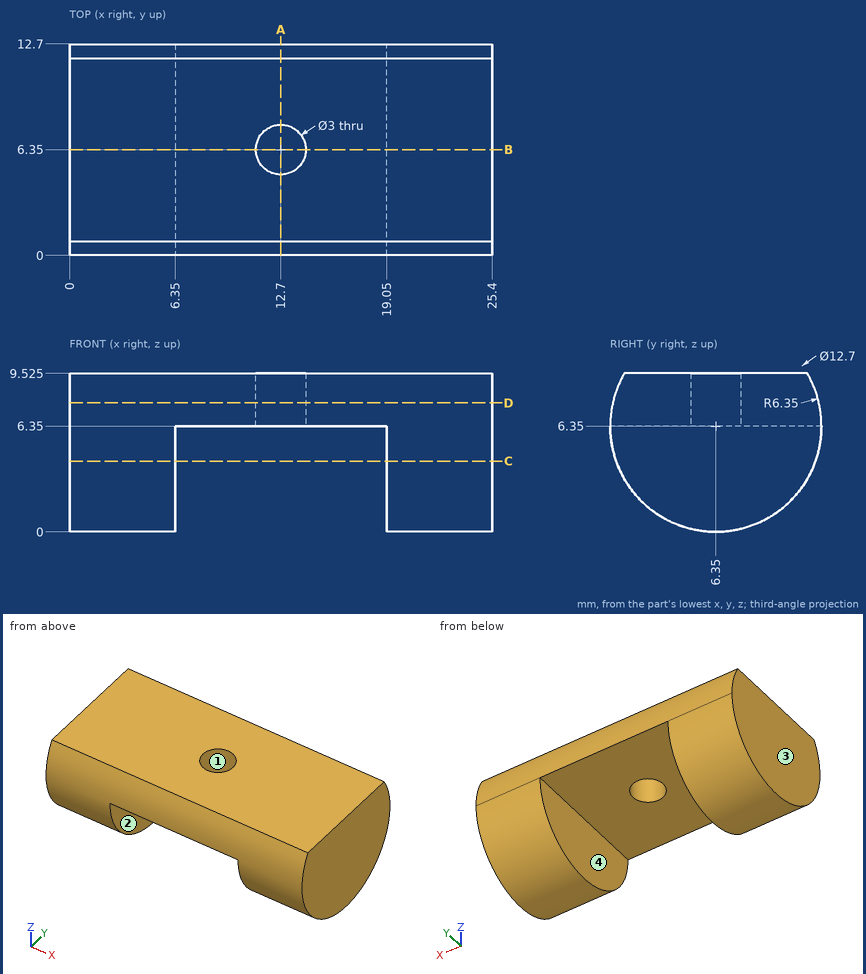
Job drawing, mm, ordinate dimensions from the low corner. One solid piece. A direction names the side the tool comes from. Give positions to 0.01 mm unless a question says otherwise; leave off trailing zeros. Loops run counter-clockwise (first coordinate to the right, second up) from the corner with the lowest first, then second, coordinate; pieces in that order, holes last. Notation, with made-up numbers: M 72,-39 L 131,-39 A35 cw 131,0 Z; hole C 26,47 d10. An arc over 180 degrees is marked long. Answer in a Markdown table with one row per item. Add a question column.
Item 1: Tool access for the marked faces 3 and 4: list every direction of +Z, -Z, +X, -X, +Y, -Y with a clear straight run to the whole face (end or side of a thin tool).
Item 2: Band-saw the part on C-C on z = 4.25. Give the cut face in (x, y).
Item 3: Drop flat-ended pins along their axis: P1, Ø1.8, axis at x = 12.7, y = 6.35, coming from the -Z side; P2, Ø1.5, axis at x = 14, y = 9.5, coming from the -Z side; P3, Ø5, axis at x = 20, z = 1.5, coming from the +Y side; P4, Ø2, axis at x = 20, z = 3.5, coming from the -Y side. Give the stop position or say it passes through.
Item 4: Band-saw the part on B-B on y = 6.35. Give the cut face in (x, z) (3 decimals), then the cut area to 3 significant figures.
Item 5: Band-saw the part on D-D on z = 7.75. Give the cut face in (x, y).
Item 6: Band-saw the part on A-A on x = 12.7. Give the cut face in (y, z) (3 decimals), then the cut area to 3 significant figures.
Item 7: Mould opens along Y. For the marked faces 1 and 2 say: +Y half, -Y half, draft (parallel to the pull), parting line (faces both ways), or undercut.
Item 8: Probe probe 1 along X at (y, z) = (5.75, 3); probe 2 along X at (y, z) = (6.35, 8.65); probe 3 along Z at (x, y) = (14.75, 9.5) (3 decimals). List the from-to ranges inside material, lowest first.
Reply:
| question | item | result |
|---|---|---|
| 1 | face 3 | +Z, -Z, -X, +Y, -Y |
| 1 | face 4 | -Z, +Y, -Y |
| 2 | outline | M 0,0.36 L 6.35,0.36 L 6.35,12.34 L 0,12.34 Z; M 19.05,0.36 L 25.4,0.36 L 25.4,12.34 L 19.05,12.34 Z |
| 3 | P1 | passes through |
| 3 | P2 | stops at z = 6.35 |
| 3 | P3 | stops at y = 12.25 |
| 3 | P4 | stops at y = 0.28 |
| 4 | outline | M 0,0 L 6.35,0 L 6.35,6.35 L 11.2,6.35 L 11.2,9.525 L 0,9.525 Z; M 14.2,6.35 L 19.05,6.35 L 19.05,0 L 25.4,0 L 25.4,9.525 L 14.2,9.525 Z |
| 4 | area | 152 mm^2 |
| 5 | outline | M 0,0.16 L 25.4,0.16 L 25.4,12.54 L 0,12.54 Z; hole C 12.7,6.35 d3 |
| 6 | outline | M 0,6.35 L 4.85,6.35 L 4.85,9.525 L 0.851,9.525 A6.35 ccw Z; M 7.85,6.35 L 12.7,6.35 A6.35 ccw 11.849,9.525 L 7.85,9.525 Z |
| 6 | area | 29.0 mm^2 |
| 7 | face 1 | undercut |
| 7 | face 2 | draft |
| 8 | probe 1 | x = 0 to 6.35, 19.05 to 25.4 |
| 8 | probe 2 | x = 0 to 11.2, 14.2 to 25.4 |
| 8 | probe 3 | z = 6.35 to 9.525 |
